For this review, use the dimensioned drawing (mm, ordinates from the lowest corner) and the shaded views. A direction names the side the tool comes from. Give positions to 0.01 mm unless a question says otherwise; leave off trailing zeros. Order: outer loops, then holes, each group sorted by start corner. A loop starts at its lowest first (then second) coordinate and runs counter-clockwise, first axis right, second up. Notation, with made-up numbers: (50.25, -38.5) -> (54.25, -38.5) arc R16 cw to (54.25, -7.5) -> close; hole circle Ø3 at (-0.75, 27.5). An arc over 180 degrees is marked (long way). Return JSON: item names as keys, results as strings.
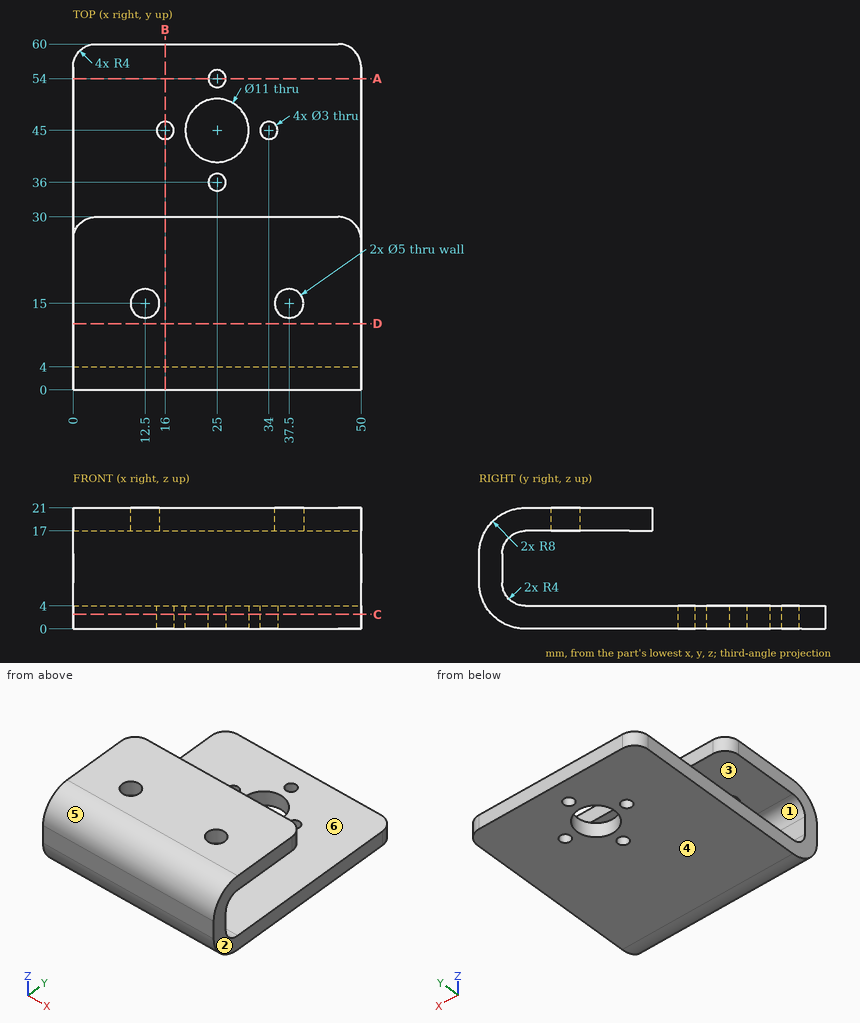
Item 1: Mouldability with a two-part tool opening along Z and no side actions: class the marked faces 3, 4, 5 and 6 as released by +Z, released by -Z, zero draft, split by the parting line, or undercut.
Result set:
{"face 3": "undercut", "face 4": "released by -Z", "face 5": "released by +Z", "face 6": "undercut"}
Item 2: For pin 1 (2.5 mm diameter, centred on x = 25, y = 36, fed in from +Z); pin 2 (3 mm diameter, centred on x = 41, y = 36, fed in from +Z); pin 3 (3 mm diameter, centred on x = 24.5, z = 19, fed in from +Y); pin 4 (1.5 mm diameter, centred on x = 36, z = 11, fed in from +Y), all flat-tipped, find the tip position at first contact; note any pin that passes through.
Result set:
{"pin 1": "passes through", "pin 2": "stops at z = 4", "pin 3": "stops at y = 30", "pin 4": "stops at y = 4"}
Item 3: Add section D-D (y = 11.5). Give the boundary of the cut face in (x, z).
Result set:
{"outline": "(0, 0) -> (50, 0) -> (50, 4) -> (0, 4) -> close; (0, 17) -> (50, 17) -> (50, 21) -> (0, 21) -> close"}
Item 4: Add section C-C (z = 2.5). Give the boundary of the cut face in (x, y), plus the area to 3 significant figures.
Result set:
{"outline": "(0, 2.19) -> (50, 2.19) -> (50, 56) arc R4 ccw to (46, 60) -> (4, 60) arc R4 ccw to (0, 56) -> close; hole circle Ø3 at (16, 45); hole circle Ø11 at (25, 45); hole circle Ø3 at (25, 36); hole circle Ø3 at (25, 54); hole circle Ø3 at (34, 45)", "area": "2,760 mm^2"}
Item 5: Add section A-A (y = 54). Give the boundary of the cut face in (x, z).
Result set:
{"outline": "(0, 0) -> (23.5, 0) -> (23.5, 4) -> (0, 4) -> close; (26.5, 0) -> (50, 0) -> (50, 4) -> (26.5, 4) -> close"}
Item 6: Wall thickness on L1, parallel to Z at x = 48.5, y = 11.5; L2, parallel to Z at x = 40.5, y = 56.5; L3, parallel to Y at x = 25, z = 3.05: over which ranges is each line inside the solid? List them lowest first. Write a range as [from, to].
Result set:
{"L1": "z = [0, 4], [17, 21]", "L2": "z = [0, 4]", "L3": "y = [1.72, 34.5], [37.5, 39.5], [50.5, 52.5], [55.5, 60]"}
Item 7: Add section B-B (x = 16). Give the boundary of the cut face in (y, z).
Result set:
{"outline": "(0, 8) arc R8 ccw to (8, 0) -> (43.5, 0) -> (43.5, 4) -> (8, 4) arc R4 cw to (4, 8) -> (4, 13) arc R4 cw to (8, 17) -> (30, 17) -> (30, 21) -> (8, 21) arc R8 ccw to (0, 13) -> close; (46.5, 0) -> (60, 0) -> (60, 4) -> (46.5, 4) -> close"}
Item 8: Machinability: for the marked faces 1 and 2, which of the approach directions +Z, -Z, +X, -X, +Y, -Y give a long, thin tool a straight path to every point of the face, cutting with its end or side? Answer none if there is none.
Result set:
{"face 1": "+X, -X, +Y", "face 2": "+Z, -Z, +X, +Y, -Y"}
